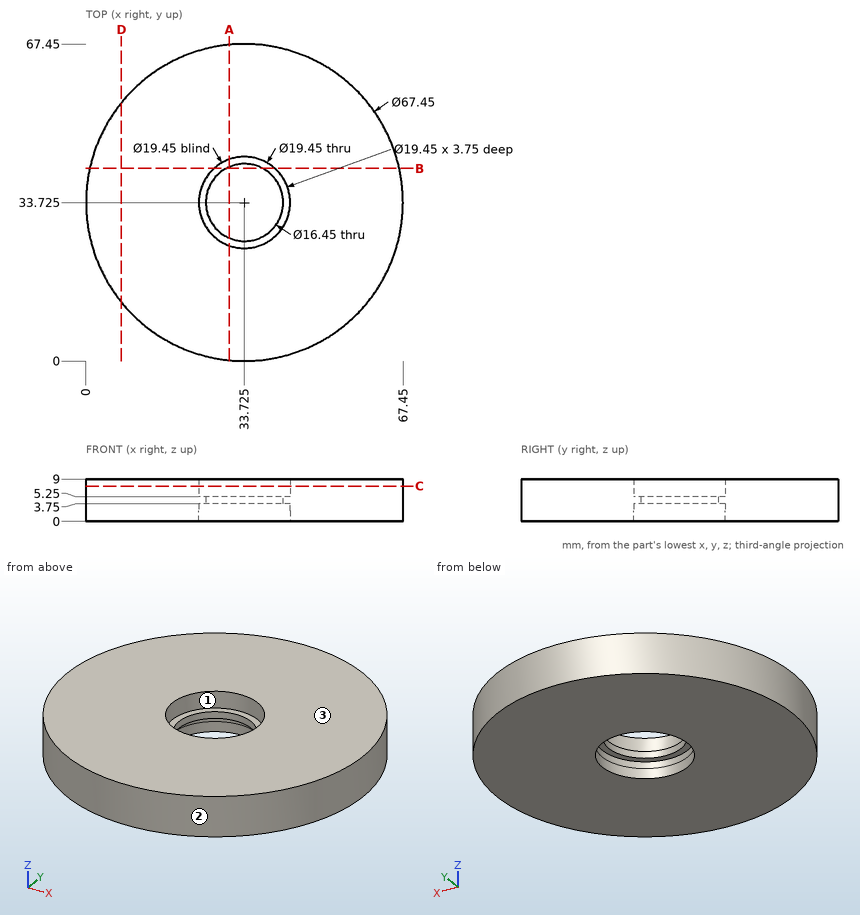
Answer from the drawing. Dimensions are ordinates in mm from the lowest x, y and z of the part. Give positions to 0.01 mm unless a question says otherwise; leave off trailing zeros. Write each loop counter-clockwise with the first axis right and the second up, starting at its lowest first coordinate (ties: lowest second). Pieces come first, ordered by that corner, then holes. Notation, with made-up numbers: (51, 46) - (94, 46) arc R14 ccw to (94, 52) - close; hole circle Ø8 at (52, 62). An arc over 180 degrees is marked (long way). Answer in a Markdown table with one row per item. Add a question column.
Item 1: Determine the mould class of the marked faces 1, 2 and 3 for opening direction Y: pulls with the +Y half, pulls with the -Y half, needs draft (parallel to the pull), parting line crosses it, or undercut.
Item 2: Section C-C, the plane z = 7.5 is taken. Write down the section's boundary in (x, y) (3 decimals).
Item 3: Flat-ended cylindrical pins translate along their axes: P1, Ø11.5, axis at x = 33.725, y = 33.725, coming from the +Z side; P2, Ø1, axis at y = 18.5, z = 4.5, coming from the +X side; P3, Ø5, axis at x = 45.5, z = 2, coming from the +Y side; P4, Ø1.5, axis at y = 36, z = 8, coming from the -X side. Find the tip coordinate at first contact, or state that the pin passes through.
Item 4: Find the intervals of material crossed by L1, parallel to Y at x = 29.5, z = 1.75; L2, parallel to X at y = 39, z = 1; L3, parallel to X at y = 33, z = 3.5, in increasing order.
Item 5: Section B-B, the plane y = 41 is taken. Write down the section's boundary in (x, z), and give its area (3 significant figures).
Item 6: Section A-A, the plane x = 30.5 is taken. Write down the section's boundary in (y, z).
Item 7: Section D-D, the plane x = 7.5 is taken. Write down the section's boundary in (y, z), and give its area (3 significant figures).
Recorded:
| question | item | result |
|---|---|---|
| 1 | face 1 | undercut |
| 1 | face 2 | parting line crosses it |
| 1 | face 3 | needs draft |
| 2 | outline | circle Ø67.45 at (33.725, 33.725); hole circle Ø19.45 at (33.725, 33.725) |
| 3 | P1 | passes through |
| 3 | P2 | stops at x = 64.07 |
| 3 | P3 | stops at y = 66.15 |
| 3 | P4 | stops at x = 0.03 |
| 4 | L1 | y = 0.27 to 24.97, 42.48 to 67.18 |
| 4 | L2 | x = 0.42 to 25.55, 41.9 to 67.03 |
| 4 | L3 | x = 0.01 to 24.03, 43.42 to 67.44 |
| 5 | outline | (0.79, 0) - (27.27, 0) - (27.27, 3.75) - (29.89, 3.75) - (29.89, 5.25) - (27.27, 5.25) - (27.27, 9) - (0.79, 9) - close; (37.56, 3.75) - (40.18, 3.75) - (40.18, 0) - (66.66, 0) - (66.66, 9) - (40.18, 9) - (40.18, 5.25) - (37.56, 5.25) - close |
| 5 | area | 484 mm2 |
| 6 | outline | (0.15, 0) - (24.55, 0) - (24.55, 3.75) - (26.16, 3.75) - (26.16, 5.25) - (24.55, 5.25) - (24.55, 9) - (0.15, 9) - close; (41.29, 3.75) - (42.9, 3.75) - (42.9, 0) - (67.3, 0) - (67.3, 9) - (42.9, 9) - (42.9, 5.25) - (41.29, 5.25) - close |
| 7 | outline | (12.52, 0) - (54.93, 0) - (54.93, 9) - (12.52, 9) - close |
| 7 | area | 382 mm2 |
